Here's how the part is built. I have some questions about the finished solid (model axes, mm). Give positions to 0.01 mm unless a question says otherwise; leave off trailing zeros. Loops run counter-clockwise (first coordinate to the right, second up) from the corner with the lowest first, then second, coordinate; pieces in that order, holes last.
Q1. Suppose I cut it at C-C (x = 89.5). List the corners of the cut face in (y, z) for me, and give its area (3 significant figures).
Q2. Suppose I cut it at B-B (z = 0). List the corners of the cut face in (x, y) for me, and give its area (3 significant figures).
Q3. I'm going to push flat-ended pins straight in: P1, Ø8, axis at x = 136.5, y = 10, coming from the +Z side; P2, Ø3, axis at y = 4.5, z = 82, coming from the -X side; P3, Ø2, axis at x = -86, y = 16.5, coming from the -Z side. Where does each tip first touch, or does it pass through?
Q4. Suppose I cut it at A-A (x = 0). List the corners of the cut face in (y, z) for me, and give its area (3 significant figures).
Q5. I need wall thicknesses on probe 1 along X at (y, z) = (8.25, 90); probe 2 along X at (y, z) = (15, 128.5); probe 3 along Z at (x, y) = (-89, 15). Which ranges of each line are inside material? Lowest first, please.
Q6. Suppose I cut it at D-D (z = 164). List the corners of the cut face in (x, y) for me, and give its area (3 significant figures).
```python
from build123d import *

# Parameters (mm, degrees)
BOSS_EXTRUDE1_DEPTH = 20
SKETCH2_R           = 7.5
CUT_EXTRUDE1_DEPTH  = 544.806031596
SKETCH3_R           = 7.5
CUT_EXTRUDE2_DEPTH  = 531.400791855
CHAMFER1_SIZE       = 10
SKETCH4_R           = 155
CUT_EXTRUDE3_DEPTH  = 341.073521463


with BuildPart() as part:
    # Sketch1 → Boss-Extrude1 (new body)
    with BuildSketch(Plane(origin=(0, 0, 0), x_dir=(1, 0, 0), z_dir=(0, 1, 0))):
        Polygon((-235, 25), (-40, 245), (40, 245), (235, 25), (235, -25), (40, -245), (-40, -245), (-235, -25), align=None)
    extrude(amount=BOSS_EXTRUDE1_DEPTH)

    # Sketch2 → Cut-Extrude1 (cut, through all)
    with BuildSketch(Plane.XY.offset(245)):
        with Locations((0, 10)):
            Circle(SKETCH2_R)
    extrude(amount=-CUT_EXTRUDE1_DEPTH, mode=Mode.SUBTRACT)

    # Sketch3 → Cut-Extrude2 (cut, through all)
    with BuildSketch(Plane(origin=(235, 0, 0), x_dir=(0, 0, -1), z_dir=(1, 0, 0))):
        with Locations((0, 10)):
            Circle(SKETCH3_R)
    extrude(amount=-CUT_EXTRUDE2_DEPTH, mode=Mode.SUBTRACT)

    # Chamfer1
    # the kernel refuses this chamfer: 10 mm, written as the material it takes off along each edge
    with BuildSketch(Plane(origin=(-235, 20, 50.71682988), x_dir=(-0.0274958766105877, -0.9996219169112968, 0), z_dir=(0, 0, -1))) as chamfer1_piece_1:
        Polygon((CHAMFER1_SIZE * 0.999621916911, -CHAMFER1_SIZE * 0.0274958766106), (-CHAMFER1_SIZE * 0.0274958766106, -CHAMFER1_SIZE * 0.999621916911), (0, 0), align=None)
    extrude(amount=101.433659759, mode=Mode.SUBTRACT)
    with BuildSketch(Plane(origin=(-22.941833496, 20, 264.245110927), x_dir=(0.7480640019059354, 0.02749587661058627, -0.6630567289620791), z_dir=(-0.6633075143158518, 0, -0.7483469392281404)), Plane(origin=(252.058166504, 20, 5.754889073), x_dir=(-0.7480640019059355, 0.02749587661058636, -0.6630567289620791), z_dir=(-0.6633075143158518, 0, 0.7483469392281404)), Plane(origin=(22.941833496, 20, -264.245110927), x_dir=(-0.7480640019059354, 0.02749587661058627, 0.6630567289620791), z_dir=(0.6633075143158519, 0, 0.7483469392281404))) as chamfer1_piece_2:
        Polygon((CHAMFER1_SIZE * 0.999621916911, CHAMFER1_SIZE * 0.0274958766106), (-CHAMFER1_SIZE * 0.0274958766106, CHAMFER1_SIZE * 0.999621916911), (0, 0), align=None)
    extrude(amount=345.414951681, mode=Mode.SUBTRACT)
    with BuildSketch(Plane(origin=(65.71682988, 20, 245), x_dir=(0, 0.027495876610586282, -0.9996219169112968), z_dir=(-1, 0, 0))) as chamfer1_piece_3:
        Polygon((CHAMFER1_SIZE * 0.999621916911, CHAMFER1_SIZE * 0.0274958766106), (-CHAMFER1_SIZE * 0.0274958766106, CHAMFER1_SIZE * 0.999621916911), (0, 0), align=None)
    extrude(amount=131.433659759, mode=Mode.SUBTRACT)
    with BuildSketch(Plane(origin=(235, 20, -50.71682988), x_dir=(-0.9996219169112968, 0.027495876610586282, 0), z_dir=(0, 0, 1))) as chamfer1_piece_4:
        Polygon((CHAMFER1_SIZE * 0.999621916911, CHAMFER1_SIZE * 0.0274958766106), (-CHAMFER1_SIZE * 0.0274958766106, CHAMFER1_SIZE * 0.999621916911), (0, 0), align=None)
    extrude(amount=101.433659759, mode=Mode.SUBTRACT)
    with BuildSketch(Plane(origin=(-65.71682988, 20, -245), x_dir=(0, -0.9996219169112968, -0.0274958766105877), z_dir=(1, 0, 0))) as chamfer1_piece_5:
        Polygon((CHAMFER1_SIZE * 0.999621916911, -CHAMFER1_SIZE * 0.0274958766106), (-CHAMFER1_SIZE * 0.0274958766106, -CHAMFER1_SIZE * 0.999621916911), (0, 0), align=None)
    extrude(amount=131.433659759, mode=Mode.SUBTRACT)
    with BuildSketch(Plane(origin=(-252.058166504, 20, -5.754889073), x_dir=(-0.020576455102926446, -0.9996219169112968, -0.018238221568502983), z_dir=(0.6633075143158518, 0, -0.7483469392281404))) as chamfer1_piece_6:
        Polygon((CHAMFER1_SIZE * 0.999621916911, -CHAMFER1_SIZE * 0.0274958766106), (-CHAMFER1_SIZE * 0.0274958766106, -CHAMFER1_SIZE * 0.999621916911), (0, 0), align=None)
    extrude(amount=345.414951681, mode=Mode.SUBTRACT)

    # Sketch4 → Cut-Extrude3 (cut, through all)
    with BuildSketch(Plane(origin=(0, 20, 0), x_dir=(1, 0, 0), z_dir=(0, 1, 0))):
        with Locations(Location((0, 0, 0), (0, 0, 270))):
            Circle(SKETCH4_R)
    extrude(amount=-CUT_EXTRUDE3_DEPTH, mode=Mode.SUBTRACT)


solid = part.part
```
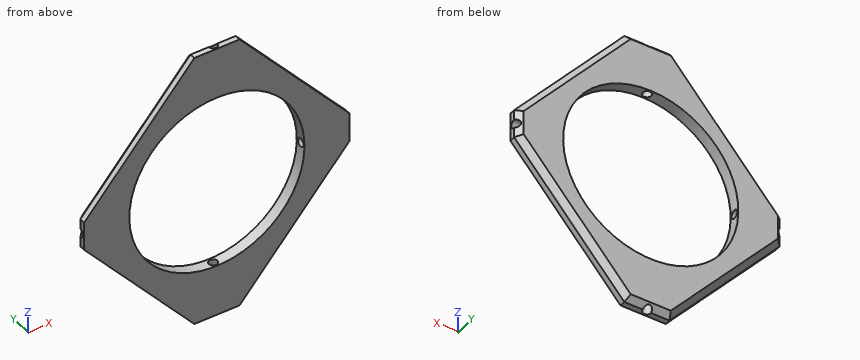
Solutions:
1. outline: (0, -189.15) - (10, -189.15) - (20, -174.08) - (20, -126.55) - (0, -126.55) - close; (0, 126.55) - (20, 126.55) - (20, 174.08) - (10, 189.15) - (0, 189.15) - close
1. area: 2,350 mm2
2. outline: (-235, 0) - (-155, 0) - (-155, 2.5) - (-235, 2.5) - close; (-227.5, 17.5) - (-155, 17.5) - (-155, 20) - (-225, 20) - close; (155, 0) - (235, 0) - (235, 2.5) - (155, 2.5) - close; (155, 17.5) - (227.5, 17.5) - (225, 20) - (155, 20) - close
2. area: 756 mm2
3. P1: stops at z = 140.64
3. P2: stops at x = -185.81
3. P3: stops at z = -185.19
4. outline: (0, -245) - (2.5, -245) - (2.5, -155) - (0, -155) - close; (0, 155) - (2.5, 155) - (2.5, 245) - (0, 245) - close; (17.5, -237.5) - (20, -235) - (20, -155) - (17.5, -155) - close; (17.5, 155) - (20, 155) - (20, 235) - (17.5, 237.5) - close
4. area: 856 mm2
5. probe 1: x = -177.39 to -126.19, 126.19 to 177.39
5. probe 2: x = -136.58 to -86.68, 86.68 to 136.58
5. probe 3: z = -182.18 to -126.9, 126.9 to 182.18
6. outline: (-111.8, 0) - (111.8, 0) - (111.8, 10) - (98.43, 20) - (-98.43, 20) - (-111.8, 10) - close; hole circle Ø15 at (0, 10)
6. area: 4,160 mm2
